Autodesk Inventor part; units mm, degrees
ref_plane "YZ Plane" through (0, 0, 0) normal (1, 0, 0) x (0, 1, 0)
ref_plane "XZ Plane" through (0, 0, 0) normal (0, 1, 0) x (-1, 0, 0)
ref_plane "XY Plane" through (0, 0, 0) normal (0, 0, 1) x (1, 0, 0)
sketch "Sketch1" plane through (0, 0, 0) normal (1, 0, 0) x (0, 1, 0)
  line L0 (0, 0) -> (190.5, 0)
  line L1 (190.5, 0) -> (190.5, -179.6034)
  line L2 (190.5, -179.6034) -> (0, -179.6034)
  line L3 (0, -179.6034) -> (0, 0)
  dimension "d0" = 190.5
  dimension "d1" = 179.6034
extrude "Extrusion1" add sketch "Sketch1" along normal blind 25.4
shell "Shell1" thickness 6.35 removed faces 1 at (25.4, 127, -119.7356)
sketch "Sketch2" plane through (6.35, 6.35, -173.2534) normal (1, 0, 0) x (0, 0, -1)
  line L0 (-32.2834, 171.45) -> (-133.8834, 171.45)
  line L1 (-133.8834, 171.45) -> (-133.8834, 6.35)
  line L2 (-133.8834, 6.35) -> (-32.2834, 6.35)
  line L3 (-32.2834, 6.35) -> (-32.2834, 171.45)
  line L4 (-166.9034, 177.8) -> (0, 177.8)
  line L5 (-166.9034, 0) -> (-166.9034, 177.8)
  point P0 (-173.2534, -6.35)
  dimension "d5" = 165.1
  dimension "d6" = 101.6
  dimension "d7" = 6.35
  dimension "d8" = 33.02
extrude "Extrusion2" cut sketch "Sketch2" against normal through all
fillet "Fillet1" radius 12.7 1 edges at (12.7, 190.5, -179.6034)
fillet "Fillet2" radius 12.7 8 edges at (12.7, 190.5, 0) (12.7, 0, 0) (12.7, 0, -179.6034) (0, 0, -89.8017) (0, 186.7803, -175.8837) (0, 190.5, -83.4517) (0, 88.9, -179.6034) (0, 95.25, 0)
properties part number "outer_casing"
Model file for the job. Use its own axes, mm. A direction names the side the tool comes from. Coordinates: 2 decimals unless noted, no trailing zeros. Order: outer loops, then holes, each group sorted by start corner. A loop starts at its lowest first (then second) coordinate and runs counter-clockwise, first axis right, second up. Notation, with made-up numbers: (27.5, 22.5) -> (50.5, 22.5) arc R27 cw to (50.5, 42.5) -> close; hole circle Ø5 at (37, 54). An arc over 180 degrees is marked (long way). Return JSON: item names as keys, results as strings. Group by question number.
Item 1: Wall check: line 1 along Z through (x, y) = (24, 14); line 2 along Y through (x, z) = (19.75, -45.5); line 3 along X through (y, z) = (125.5, -15). Give the ranges that are in metal, low to high. Write a range as [from, to].
Item 2: Pull direction Y, two halves, no side cores. Call faces 1 (the cylindrical face through (19.139, 186.681, -175.982)), 2 (the cylindrical face through (3.62, 96.41, -3.82)), 3 (the flat face through (3, 177.8, -91)), 4 (the flat face through (16, 96, -173.253)): pulls with the +Y half, pulls with the -Y half, needs draft (parallel to the pull), parting line crosses it, or undercut.
Item 3: Flat gauge pins, fed straight in: P1, Ø5, axis at x = 2.5, z = -98.5, coming from the -Y side; P2, Ø9.5, axis at x = 16, y = 61, coming from the +Z side; P3, Ø2, axis at x = 10, y = 37, coming from the +Z side; P4, Ø7, axis at x = 2, z = -111, coming from the +Y side. Where does each tip first touch, or does it go through?
Item 4: Saw through at A-A on y = 175. Write the cut outline in (x, z).
Item 5: Tool access for faces 5 (the flat face through (6.35, 94, -144)), 6 (the flat face through (3, 96, -39.37)), 7 (the flat face through (19, 94, 0)): list every direction of +Z, -Z, +X, -X, +Y, -Y with a clear straight run to the whole face (end or side of a thin tool).
Item 6: Saw through at D-D on x = 17.75. Write the cut outline in (y, z), then the cut area to 3 significant figures.
Item 7: Saw through at B-B on z = -151. Write the cut outline in (x, y).
Values found:
{
 "1": {"line 1": "z = [-179.6, -173.25], [-6.35, 0]", "line 2": "y = [0, 6.35], [184.15, 190.5]", "line 3": "x = [0, 6.35]"},
 "2": {"face 1": "pulls with the +Y half", "face 2": "needs draft", "face 3": "undercut", "face 4": "undercut"},
 "3": {"P1": "stops at y = 2.6", "P2": "stops at z = 0", "P3": "stops at z = -0.11", "P4": "stops at y = 188.26"},
 "4": {"outline": "(0, -166.9) arc R12.7 ccw to (12.7, -179.6) -> (25.4, -179.6) -> (25.4, -173.25) -> (6.35, -173.25) -> (6.35, -140.97) -> (0, -140.97) -> close; (0, -39.37) -> (6.35, -39.37) -> (6.35, -6.35) -> (25.4, -6.35) -> (25.4, 0) -> (12.7, 0) arc R12.7 ccw to (0, -12.7) -> close"},
 "5": {"face 5": "+X", "face 6": "+X, -X", "face 7": "+Z, +X, -X, +Y, -Y"},
 "6": {"outline": "(0, -166.9) arc R12.7 ccw to (12.7, -179.6) -> (177.8, -179.6) arc R12.7 ccw to (190.5, -166.9) -> (190.5, -12.7) arc R12.7 ccw to (177.8, 0) -> (12.7, 0) arc R12.7 ccw to (0, -12.7) -> close; hole (6.35, -173.25) -> (184.15, -173.25) -> (184.15, -6.35) -> (6.35, -6.35) -> close", "area": "4,400 mm2"},
 "7": {"outline": "(0, 12.7) arc R12.7 ccw to (12.7, 0) -> (25.4, 0) -> (25.4, 6.35) -> (6.35, 6.35) -> (6.35, 184.15) -> (25.4, 184.15) -> (25.4, 190.5) -> (12.7, 190.5) arc R12.7 ccw to (0, 177.8) -> close"}
}
